from build123d import *

# Parameters (mm, degrees)
SKETCH1_R           = 7.0231
SKETCH1_R_2         = 7.0104
BOSS_EXTRUDE2_DEPTH = 9.906
SKETCH2_R           = 9.9822
SKETCH2_R_2         = 4.98475
BOSS_EXTRUDE3_DEPTH = 1.9812
SKETCH4_R           = 9.9822
SKETCH4_R_2         = 7.0231
BOSS_EXTRUDE4_DEPTH = 9.906
SKETCH5_R           = 8.0264
CUT_EXTRUDE1_DEPTH  = 5.2324
CUT_EXTRUDE2_DEPTH  = 5.5372
SKETCH7_R           = 1.9685
CUT_EXTRUDE3_DEPTH  = 12.7
CUT_EXTRUDE4_DEPTH  = 4.064


with BuildPart() as part:
    # Sketch1 → Boss-Extrude2 (new body)
    # profile 1 of 2: a face of its own
    with BuildSketch(Plane.XY):
        with BuildLine():
            Line((-7.77875, 14.0589), (-5.59435, 4.245842871))
            ThreePointArc((-5.59435, 4.245842871), (2.239894431, 6.65633582), (7.0231, 0))
            ThreePointArc((7.0231, 0), (2.239894431, -6.65633582), (-5.59435, -4.245842871))
            Line((-5.59435, -4.245842871), (-8.03275, -16.9545))
            Line((-8.03275, -16.9545), (-12.68095, -16.9545))
            Line((-12.68095, -16.9545), (-12.68095, -21.9583))
            Line((-12.68095, -21.9583), (26.84145, -21.9583))
            Line((26.84145, -21.9583), (26.84145, -25.0063))
            Line((26.84145, -25.0063), (50.69205, -25.0063))
            Line((50.69205, -25.0063), (53.38445, -19.7231))
            Line((53.38445, -19.7231), (56.55945, -19.7231))
            ThreePointArc((56.55945, -19.7231), (60.50132397, 1.056607323), (45.49775, 15.9639))
            Line((45.49775, 15.9639), (18.29435, 15.9639))
            Line((18.29435, 15.9639), (12.45235, 19.0119))
            Line((12.45235, 19.0119), (5.49275, 19.0119))
            Line((5.49275, 19.0119), (3.460028891, 11.9761))
            Line((3.460028891, 11.9761), (-3.460028891, 11.9761))
            Line((-3.460028891, 11.9761), (-5.49275, 19.0119))
            Line((-5.49275, 19.0119), (-12.68095, 19.0119))
            Line((-12.68095, 19.0119), (-12.68095, 14.0589))
            Line((-12.68095, 14.0589), (-7.77875, 14.0589))
        make_face()
        with BuildLine():
            ThreePointArc((25.235083599, -18.8595), (23.774583599, -17.399), (25.235083599, -15.9385))
            Line((25.235083599, -15.9385), (48.298283599, -15.9385))
            ThreePointArc((48.298283599, -15.9385), (49.758783599, -17.399), (48.298283599, -18.8595))
            Line((48.298283599, -18.8595), (25.235083599, -18.8595))
        make_face(mode=Mode.SUBTRACT)
        with BuildLine():
            ThreePointArc((27.368683599, -12.8397), (19.469283599, -4.9403), (27.368683599, 2.9591))
            Line((27.368683599, 2.9591), (46.164683599, 2.9591))
            ThreePointArc((46.164683599, 2.9591), (54.064083599, -4.9403), (46.164683599, -12.8397))
            Line((46.164683599, -12.8397), (27.368683599, -12.8397))
        make_face(mode=Mode.SUBTRACT)
        with BuildLine():
            ThreePointArc((25.235083599, 6.5405), (23.774583599, 8.001), (25.235083599, 9.4615))
            Line((25.235083599, 9.4615), (48.298283599, 9.4615))
            ThreePointArc((48.298283599, 9.4615), (49.758783599, 8.001), (48.298283599, 6.5405))
            Line((48.298283599, 6.5405), (25.235083599, 6.5405))
        make_face(mode=Mode.SUBTRACT)
    # profile 2 of 2: a face of its own
    with BuildSketch(Plane.XY):
        Circle(SKETCH1_R)
        Circle(SKETCH1_R_2, mode=Mode.SUBTRACT)
    extrude(amount=BOSS_EXTRUDE2_DEPTH)

    # Sketch2 → Boss-Extrude3 (add)
    with BuildSketch(Plane(origin=(0, 0, 0), x_dir=(-1, 0, 0), z_dir=(0, 0, -1))):
        with Locations(Location((0, 0, 0), (0, 0, 308.91150739))):
            Circle(SKETCH2_R)
        Circle(SKETCH2_R_2, mode=Mode.SUBTRACT)
    extrude(amount=BOSS_EXTRUDE3_DEPTH)

    # Sketch4 → Boss-Extrude4 (add)
    with BuildSketch(Plane.XY):
        with Locations(Location((0, 0, 0), (0, 0, 231.08849261))):
            Circle(SKETCH4_R)
        Circle(SKETCH4_R_2, mode=Mode.SUBTRACT)
    extrude(amount=BOSS_EXTRUDE4_DEPTH)

    # Sketch5 → Cut-Extrude1 (cut)
    with BuildSketch(Plane(origin=(0, 0, -1.9812), x_dir=(-1, 0, 0), z_dir=(0, 0, -1))):
        Circle(SKETCH5_R)
    extrude(amount=-CUT_EXTRUDE1_DEPTH, mode=Mode.SUBTRACT)

    # Sketch6 → Cut-Extrude2 (cut)
    with BuildSketch(Plane(origin=(0, 0, 0), x_dir=(-1, 0, 0), z_dir=(0, 0, -1))):
        with BuildLine():
            Line((-46.164683599, 2.9591), (-59.816731187, 2.9591))
            ThreePointArc((-59.816731187, 2.9591), (-61.500748438, -4.894234845), (-60.325858759, -12.8397))
            Line((-60.325858759, -12.8397), (-46.164683599, -12.8397))
            Line((-46.164683599, -12.8397), (-46.164683599, 2.9591))
        make_face()
    extrude(amount=-CUT_EXTRUDE2_DEPTH, mode=Mode.SUBTRACT)

    # Sketch7 → Cut-Extrude3 (cut)
    with BuildSketch(Plane.XZ.offset(21.9583)):
        with Locations(Location((-8.93445, 4.953, 0), (0, 0, 270))):
            Circle(SKETCH7_R)
        with Locations(Location((17.43075, 4.953, 0), (0, 0, 270))):
            Circle(SKETCH7_R)
    extrude(amount=-CUT_EXTRUDE3_DEPTH, mode=Mode.SUBTRACT)

    # Sketch8 → Cut-Extrude4 (cut)
    with BuildSketch(Plane(origin=(0, 0, 0), x_dir=(-1, 0, 0), z_dir=(0, 0, -1))):
        with BuildLine():
            Line((-48.298283599, 11.303), (-25.235083599, 11.303))
            ThreePointArc((-25.235083599, 11.303), (-21.933083599, 8.001), (-25.235083599, 4.699))
            Line((-25.235083599, 4.699), (-48.298283599, 4.699))
            ThreePointArc((-48.298283599, 4.699), (-51.600283599, 8.001), (-48.298283599, 11.303))
        make_face()
        with BuildLine():
            Line((-48.298283599, -14.097), (-25.235083599, -14.097))
            ThreePointArc((-25.235083599, -14.097), (-21.933083599, -17.399), (-25.235083599, -20.701))
            Line((-25.235083599, -20.701), (-48.298283599, -20.701))
            ThreePointArc((-48.298283599, -20.701), (-51.600283599, -17.399), (-48.298283599, -14.097))
        make_face()
    extrude(amount=-CUT_EXTRUDE4_DEPTH, mode=Mode.SUBTRACT)


solid = part.part
Work out the finished part from the listing and answer in its coordinate system (mm). A direction names the side the tool comes from. Round coordinates to 2 decimals unless told otherwise and drop trailing zeros. Write each loop counter-clockwise with the first axis right and the second up, starting at its lowest first coordinate (ties: lowest second). Pieces come first, ordered by that corner, then holes.
1) The mould has two halves that part along Y. Classify faces 1 (the flat face through (32, 15.964, 5)), 2 (the flat face through (55, -19.723, 5)), 3 (the flat face through (56, -5, 5.537)): pulls with the +Y half, pulls with the -Y half, needs draft (parallel to the pull), parting line crosses it, or undercut.
2) Given pin 1 Ø6.5 at (x, z) = (40.5, 6.5) entering from +Y; pin 2 Ø10 at (x, y) = (17, 13.5) entering from -Z; pin 3 Ø3 at (y, z) = (-17.5, 7) entering from +X, each flat-ended and moving along its own axis, determine where each tip first touches the part or whether it passes through.
3) A tool of negligible diameter and unlimited length cuts with its end or side. For faces 4 (the cylindrical face through (-6.983, -18.845, 5.209)), 5 (the flat face through (-3, -7, 3.251)), 6 (the cylindrical face through (23.775, 7.969, 6.944)), 7 (the flat face through (-11.4, -16.954, 4.9)), from which of +Z, -Z, +X, -X, +Y, -Y can it reach the whole face along a straight path? Write none if from no direction.
4) A cutting plane is placed at B-B (x = 0). Give the vertices of the cut face in (y, z).
5) Straight lines are drawn through the part: line 1 (Y direction, x = 30, z = 1.5); line 2 (Y direction, x = 0, z = 4.75); line 3 (Z direction, x = 14, y = 2.5). For each, find the intervals that lie inside material, in ascending order.
6) A cutting plane is placed at A-A (z = 1.25). Give the number of separate pieces and of enclosed holes in the cut face, plus the area to 3 significant figures.
7) A cutting plane is placed at C-C (y = 13). Give the vertices of the cut face in (x, z), plus the area to 3 significant figures.
Completed:
1. face 1: pulls with the +Y half
1. face 2: pulls with the -Y half
1. face 3: undercut
2. pin 1: stops at y = 15.96
2. pin 2: stops at z = 0
2. pin 3: stops at x = 58.98
3. face 4: -Y
3. face 5: -Z
3. face 6: +Z, -Z
3. face 7: +Z, -Z, -X
4. outline: (-21.96, 0) - (-9.98, 0) - (-9.98, -1.98) - (-8.03, -1.98) - (-8.03, 3.25) - (-7.01, 3.25) - (-7.01, 9.91) - (-21.96, 9.91) - close; (7.01, 3.25) - (8.03, 3.25) - (8.03, -1.98) - (9.98, -1.98) - (9.98, 0) - (11.98, 0) - (11.98, 9.91) - (7.01, 9.91) - close
5. line 1: y = -25.01 to -20.7, -14.1 to -12.84, 2.96 to 4.7, 11.3 to 15.96
5. line 2: y = -21.96 to -7.01, 7.01 to 11.98
5. line 3: z = 0 to 9.91
6. separate pieces: 1
6. enclosed holes: 3
6. area: 1,430 mm2
7. outline: (-7.54, 0) - (-3.76, 0) - (-3.76, 9.91) - (-7.54, 9.91) - close; (3.76, 0) - (51.68, 0) - (51.68, 9.91) - (3.76, 9.91) - close
7. area: 512 mm2
